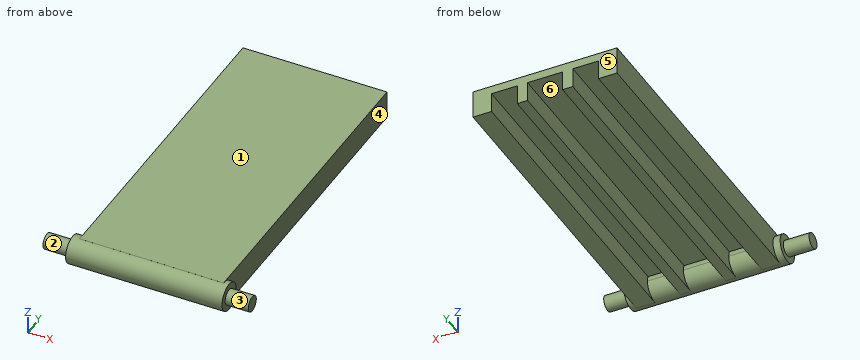
from build123d import *

# Parameters (mm, degrees)
F1_DEPTH  = 310
F0_W      = 34
F0_H      = 8
F2_DEPTH  = 250
F3_DEPTH  = 310
F0_W_2    = 25
F4_DEPTH  = 309.9
F5_R      = 13.5
F6_DEPTH  = 76
F7_R      = 7.5823100612
F8_DEPTH  = 325
F9_DEPTH  = 177
F10_DEPTH = 162.7
F11_DEPTH = 154.5


with BuildPart() as f1:
    # F0 (on Front) → F1 (new body)
    with BuildSketch(Plane.XZ):
        Polygon((70.9833226877, 8), (52.9833226877, 8), (52.9833226877, 0), (52.9833226877, -19.1598301306), (70.9833226877, -19.1598301306), (70.9833226877, 3.8401698694), align=None)
    extrude(amount=F1_DEPTH)



with BuildPart() as f1b:
    # F0 (on Front) → F1, piece 2 (new body)
    with BuildSketch(Plane.XZ):
        Polygon((-69.0166773123, -19.1598301306), (-51.0166773123, -19.1598301306), (-51.0166773123, 0), (-51.0166773123, 8), (-69.0166773123, 8), (-69.0166773123, 3.8401698694), align=None)
    extrude(amount=F1_DEPTH)


with BuildPart() as f2:
    # F0 (on Front) → F2 (new body)
    with BuildSketch(Plane.XZ):
        with Locations((0.9833226877, 4)):
            Rectangle(F0_W, F0_H)
    extrude(amount=F2_DEPTH)

    # F0 (on Front) → F3 (join)
    with BuildSketch(Plane.XZ):
        Polygon((-26.0166773123, 8), (-26.0166773123, 0), (-26.0166773123, -19.1598301306), (-16.0166773123, -19.1598301306), (-16.0166773123, 0), (-16.0166773123, 8), align=None)
        Polygon((27.9833226877, 8), (17.9833226877, 8), (17.9833226877, 0), (17.9833226877, -19.1598301306), (27.9833226877, -19.1598301306), (27.9833226877, 0), align=None)
    extrude(amount=F3_DEPTH)


with BuildPart() as f4:
    # F0 (on Front) → F4 (new body)
    with BuildSketch(Plane.XZ):
        with Locations((-38.5166773123, 4)):
            Rectangle(F0_W_2, F0_H)
    extrude(amount=F4_DEPTH)


with BuildPart() as f4b:
    # F0 (on Front) → F4, piece 2 (new body)
    with BuildSketch(Plane.XZ):
        with Locations((40.4833226877, 4)):
            Rectangle(F0_W_2, F0_H)
    extrude(amount=F4_DEPTH)


with BuildPart() as f4c:
    # F0 (on Front) → F4, piece 3 (new body)
    with BuildSketch(Plane.XZ):
        with Locations((0.9833226877, 4)):
            Rectangle(F0_W, F0_H)
    extrude(amount=F4_DEPTH)


with BuildPart() as f1_1:
    add(f1.part)

    add(f1b.part)  # F6 merges F1b

    add(f2.part)  # F6 merges F2

    add(f4.part)  # F6 merges F4

    add(f4b.part)  # F6 merges F4b

    add(f4c.part)  # F6 merges F4c
    # F5 (on Right) → F6 (join, symmetric)
    with BuildSketch(Plane.YZ):
        with Locations((-309.2783357923, -5.516671653)):
            Circle(F5_R)
    extrude(amount=F6_DEPTH, both=True)

    # F7 (on face) → F8 (cut)
    with BuildSketch(Plane.YZ.offset(76)):
        with Locations((-309.2783357923, -5.516671653)):
            Circle(F7_R)
    extrude(amount=-F8_DEPTH, mode=Mode.SUBTRACT)

    # F7 (on face) → F9 (join, symmetric)
    with BuildSketch(Plane.YZ.offset(76)):
        with Locations((-309.2783357923, -5.516671653)):
            Circle(F7_R)
    extrude(amount=F9_DEPTH, both=True)

    # F10 (add): a face of the model
    f10_faces = [f1_1.faces().sort_by_distance(p)[0] for p in [
        (253, -309.2783357923, -5.516671653),
    ]]
    extrude(f10_faces, amount=-F10_DEPTH)

    # F11 (cut): a face of the model
    f11_faces = [f1_1.faces().sort_by_distance(p)[0] for p in [
        (253, -309.2783357923, -5.516671653),
    ]]
    extrude(f11_faces, amount=-F11_DEPTH, mode=Mode.SUBTRACT)


solid = f1_1.part
Input: part model. Units: mm. Frame: model coordinates. Face numbers are marked on the shaded views. A direction names the side the tool comes from. Coordinates: 2 decimals unless noted, no trailing zeros. Loops run counter-clockwise (first coordinate to the right, second up) from the corner with the lowest first, then second, coordinate; pieces in that order, holes last. Notation, with made-up numbers: (32.5, 62.5) - (88.5, 62.5) arc R33 ccw to (88.5, 94.5) - close; hole circle Ø7 at (89, 72). An arc over 180 degrees is marked (long way). Answer in a Markdown table with one row per item. Add a question column.
Item 1: Access query for the marked faces 1, 2 and 3. Directions: +Z, -Z, +X, -X, +Y, -Y. A direction counts if a zero-diameter tool reaches every point of the face in a straight line with its end or side. Return the directions, or none.
Item 2: Contact query for flat-ended pins moving along their axis: P1, Ø10, axis at x = 7, y = -190.5, coming from the -Z side; P2, Ø13.5, axis at y = -199.5, z = -11.5, coming from the -X side; P3, Ø10, axis at y = -101, z = -12.5, coming from the +X side. Output: stop coordinate, or through.
Item 3: Section query C-C on z = -9. Return the cut outline in (x, y), then the cut area to 3 significant figures.
Item 4: Line query: line 1 along X through (y, z) = (-36, -11.25); line 2 along X through (y, z) = (-75, 6); line 3 along Z through (x, y) = (9, -226.5). Output: solid intervals per line, ascending. Write a range as [from, to].
Item 5: Section query A-A on y = -172. Return the cut outline in (x, z).
Item 6: Mould query, pull axis X, two halves, no side actions, for the marked faces 4, 5 and 6. Classes: released by +X, released by -X, zero draft, split by the parting line, or undercut.
Recorded:
| question | item | result |
|---|---|---|
| 1 | face 1 | +Z, +X, -X, +Y, -Y |
| 1 | face 2 | -X |
| 1 | face 3 | +X |
| 2 | P1 | z = 0 |
| 2 | P2 | x = -69.02 |
| 2 | P3 | x = 70.98 |
| 3 | outline | (-101, -316.01) - (-76, -316.01) - (-76, -322.32) - (76, -322.32) - (76, -316.01) - (98.5, -316.01) - (98.5, -302.54) - (76, -302.54) - (76, -296.24) - (70.98, -296.24) - (70.98, 0) - (52.98, 0) - (52.98, -296.24) - (27.98, -296.24) - (27.98, 0) - (17.98, 0) - (17.98, -296.24) - (-16.02, -296.24) - (-16.02, 0) - (-26.02, 0) - (-26.02, -296.24) - (-51.02, -296.24) - (-51.02, 0) - (-69.02, 0) - (-69.02, -296.24) - (-76, -296.24) - (-76, -302.54) - (-101, -302.54) - close |
| 3 | area | 21,200 mm^2 |
| 4 | line 1 | [-69.02, -51.02], [-26.02, -16.02], [17.98, 27.98], [52.98, 70.98] |
| 4 | line 2 | [-69.02, 70.98] |
| 4 | line 3 | [0, 8] |
| 5 | outline | (-69.02, -19.16) - (-51.02, -19.16) - (-51.02, 0) - (-26.02, 0) - (-26.02, -19.16) - (-16.02, -19.16) - (-16.02, 0) - (17.98, 0) - (17.98, -19.16) - (27.98, -19.16) - (27.98, 0) - (52.98, 0) - (52.98, -19.16) - (70.98, -19.16) - (70.98, 8) - (-69.02, 8) - close |
| 6 | face 4 | released by +X |
| 6 | face 5 | zero draft |
| 6 | face 6 | undercut |
